Autodesk Fusion 360 part; units mm, degrees
sketch "Szkic1" plane through (0, 0, 0) normal (0, 0, 1) x (1, 0, 0)
  line L0 (-39.0522, 48.0519) -> (259.5478, 48.0519)
  line L1 (259.5478, 48.0519) -> (259.5478, -41.9481)
  line L2 (259.5478, -41.9481) -> (-39.0522, -41.9481)
  line L3 (-39.0522, -41.9481) -> (-39.0522, 48.0519)
  line L4 (-44.0522, 53.0519) -> (263.9478, 53.0519)
  line L5 (263.9478, 53.0519) -> (263.9478, -46.9481)
  line L6 (263.9478, -46.9481) -> (-44.0522, -46.9481)
  line L7 (-44.0522, -46.9481) -> (-44.0522, 53.0519)
  line L8 (118.5478, -41.9481) -> (106.5478, -41.9481)
  line L9 (106.5478, -41.9481) -> (106.5478, -46.9481)
  line L10 (106.5478, -46.9481) -> (118.5478, -46.9481)
  line L11 (118.5478, -46.9481) -> (118.5478, -41.9481)
  dimension "d1" = 298.6
  dimension "d2" = 90
  dimension "d3" = 308
  dimension "d4" = 100
  dimension "d5" = 5
  dimension "d6" = 5
  dimension "d7" = 141
  dimension "d8" = 12
extrude "Wyciągnięcie proste1" add sketch "Szkic1" along normal blind 5 contours L0 L1 L2 L3 L4 L5 L6 L7 L9 L11
extrude "Wyciągnięcie proste2" add sketch "Szkic1" along normal blind 2 contours L0 L1 L2 L3 L8
extrude "Wyciągnięcie proste3" add sketch "Szkic1" along normal blind 2 contours L2 L6 L8 L9 L10 L11
extrude "Wyciągnięcie proste4" add 1 faces at (60.2811, 51.3852, 5) along direction (0, 0, 1) blind 5
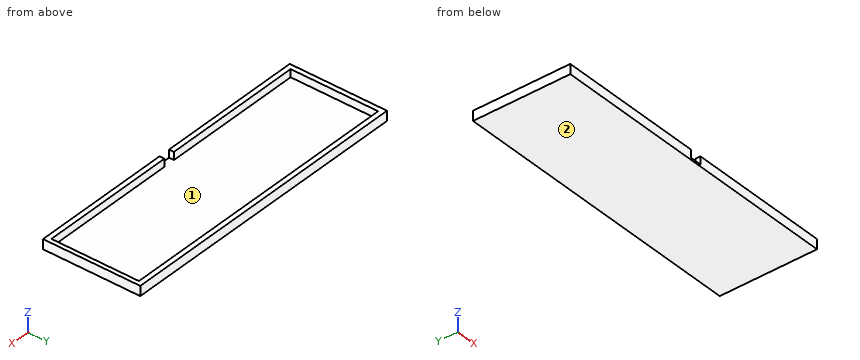
Geometry: final body of the model. Coordinates: model frame, mm. Face numbers are marked on the shaded views. Round coordinates to 2 decimals unless told otherwise and drop trailing zeros. Write each loop counter-clockwise with the first axis right and the second up, starting at its lowest first coordinate (ties: lowest second). Pieces come first, ordered by that corner, then holes.
Item 1: Section query D-D (x = 6.5). Return loops of the section in (y, z).
Item 2: Section query B-B (y = -25). Return loops of the section in (x, z).
Item 3: Section query A-A (x = 112.5). Return loops of the section in (y, z), plus the area to 3 significant figures.
Item 4: Material intervals for L1, parallel to X at y = 44.5, z = 4; L2, parallel to Y at x = 150, z = 6.25; L3, parallel to Z at x = 235, y = 41, sorted ascending.
Item 5: Section query C-C (z = 4.5). Return loops of the section in (x, y).
Item 6: Pin query (flat end, axial travel): P1, Ø4, axis at x = 3, y = -17.5, coming from the +Z side. Return the tip coordinate at first contact, or that it passes through.
Item 7: Mould query, pull axis Y, two halves, no side actions, for the marked faces 1 and 2. Classes: +Y half, -Y half, draft (parallel to the pull), parting line (faces both ways), or undercut.
Completed:
1. outline: (-46.95, 0) - (53.05, 0) - (53.05, 10) - (48.05, 10) - (48.05, 2) - (-41.95, 2) - (-41.95, 10) - (-46.95, 10) - close
2. outline: (-44.05, 0) - (263.95, 0) - (263.95, 10) - (259.55, 10) - (259.55, 2) - (-39.05, 2) - (-39.05, 10) - (-44.05, 10) - close
3. outline: (-46.95, 0) - (53.05, 0) - (53.05, 10) - (48.05, 10) - (48.05, 2) - (-46.95, 2) - close
3. area: 240 mm2
4. L1: x = -44.05 to -39.05, 259.55 to 263.95
4. L2: y = -46.95 to -41.95, 48.05 to 53.05
4. L3: z = 0 to 2
5. outline: (-44.05, -46.95) - (106.55, -46.95) - (106.55, -41.95) - (-39.05, -41.95) - (-39.05, 48.05) - (259.55, 48.05) - (259.55, -41.95) - (118.55, -41.95) - (118.55, -46.95) - (263.95, -46.95) - (263.95, 53.05) - (-44.05, 53.05) - close
6. P1: stops at z = 2
7. face 1: undercut
7. face 2: draft
